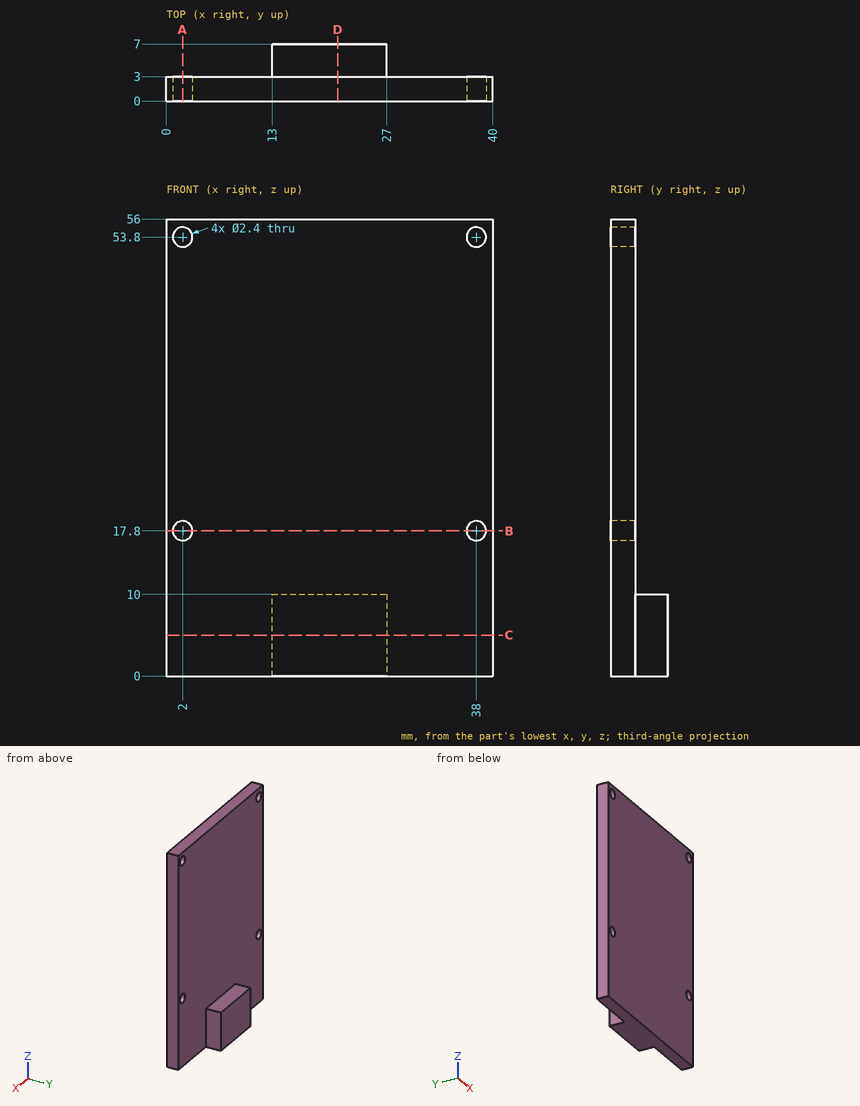
Input: dimensioned drawing with shaded views. Units: mm. Origin: part minimum x, y, z. Give positions to 0.01 mm unless a question says otherwise; leave off trailing zeros. Write each loop counter-clockwise with the first axis right and the second up, starting at its lowest first coordinate (ties: lowest second). Pieces come first, ordered by that corner, then holes.
1. Pin query (flat end, axial travel): P1, Ø4, axis at x = 38, z = 53.8, coming from the +Y side; P2, Ø2, axis at y = 5, z = 5, coming from the -X side. Return the tip coordinate at first contact, or that it passes through.
2. Section query A-A, the plane x = 2. Return loops of the section in (y, z).
3. Section query D-D, the plane x = 21. Return loops of the section in (y, z).
4. Line query: probe 1 along X at (y, z) = (0.65, 17.8); probe 2 along Z at (x, y) = (2, 1.9); probe 3 along Y at (x, z) = (15, 31.5). Output: solid intervals per line, ascending.
5. Section query C-C, the plane z = 5. Return loops of the section in (x, y), then the cut area to 3 significant figures.
6. Section query B-B, the plane z = 17.8. Return loops of the section in (x, y).
Computed:
1. P1: stops at y = 3
1. P2: stops at x = 13
2. outline: (0, 0) - (3, 0) - (3, 16.6) - (0, 16.6) - close; (0, 19) - (3, 19) - (3, 52.6) - (0, 52.6) - close; (0, 55) - (3, 55) - (3, 56) - (0, 56) - close
3. outline: (0, 0) - (7, 0) - (7, 10) - (3, 10) - (3, 56) - (0, 56) - close
4. probe 1: x = 0 to 0.8, 3.2 to 36.8, 39.2 to 40
4. probe 2: z = 0 to 16.6, 19 to 52.6, 55 to 56
4. probe 3: y = 0 to 3
5. outline: (0, 0) - (40, 0) - (40, 3) - (27, 3) - (27, 7) - (13, 7) - (13, 3) - (0, 3) - close
5. area: 176 mm2
6. outline: (0, 0) - (0.8, 0) - (0.8, 3) - (0, 3) - close; (3.2, 0) - (36.8, 0) - (36.8, 3) - (3.2, 3) - close; (39.2, 0) - (40, 0) - (40, 3) - (39.2, 3) - close
